Input: part model. Units: mm. Frame: model coordinates. A direction names the side the tool comes from. Coordinates: 2 decimals unless noted, no trailing zeros. Write each loop counter-clockwise with the first axis right and the second up, starting at its lowest first coordinate (ties: lowest second). Pieces come first, ordered by that corner, then holes. Notation, with made-up numbers: M -10.75,23.5 L 2.25,23.5 A16 cw 2.25,52.5 Z; hole C -26.5,-38 d6. An arc over 180 degrees is marked long. Write each question's results on one line, items separated by ' | '. Start each with the question number.
1. Section query B-B, the plane x = -105. Output: boundary loops of the cut face in (y, z), and give its area (3 significant figures).
2. Section query C-C, the plane y = 85. Output: boundary loops of the cut face in (x, z).
3. First-contact query: pin 1 (4 mm diameter, centred on x = 100.5, y = 92, fed in from +Z). Flat tip, straight axial feed; report the tip coordinate or a pass-through.
4. Section query A-A, the plane z = 89.5. Output: boundary loops of the cut face in (x, y).
5. Pull-direction query (X, two-part tool) for faces 3 (the flat face through (-96, -584, 127)), 4 (the flat face through (1219.2, -9, 63)), 5 (the flat face through (-16, 8, 25.4)), 6 (the flat face through (-1219.2, -9, 63)); classes: +X half, -X half, draft (parallel to the pull), parting line (faces both ways), or undercut.
6. Ray query, probe 1 along X at (y, z) = (248, 63); probe 2 along Y at (x, z) = (-781.5, 90.5); probe 3 along Z at (x, y) = (-842, 26). Return the intervals inside material, ascending.
7. Set-up query: faces 1 (the flat face through (-17, -660.4, 63)), 2 (the flat face through (-16, -558.8, 75)). Return all of +Z, -Z, +X, -X, +Y, -Y with unobstructed straight access to the full face (end or side cutting, diameter ignored); none if empty.
```python
from build123d import *

# Parameters (mm, degrees)
F0_W     = 2438.4
F0_H     = 1320.8
F0_W_2   = 2235.2
F0_H_2   = 1117.6
F1_DEPTH = 25.4
F2_W     = 2438.4
F2_H     = 1320.8
F2_W_2   = 2235.2
F2_H_2   = 1117.6
F3_DEPTH = 101.6


with BuildPart() as f1:
    # F0 (on Top) → F1 (new body)
    with BuildSketch(Plane.XY):
        Rectangle(F0_W, F0_H)
        Rectangle(F0_W_2, F0_H_2, mode=Mode.SUBTRACT)
        Rectangle(F0_W_2, F0_H_2)
    extrude(amount=F1_DEPTH)

    # F2 (on face) → F3 (join)
    with BuildSketch(Plane.XY.offset(25.4)):
        Rectangle(F2_W, F2_H)
        Rectangle(F2_W_2, F2_H_2, mode=Mode.SUBTRACT)
    extrude(amount=F3_DEPTH)


solid = f1.part
```
Answer:
1) outline: M -660.4,0 L 660.4,0 L 660.4,127 L 558.8,127 L 558.8,25.4 L -558.8,25.4 L -558.8,127 L -660.4,127 Z | area: 54,200 mm^2
2) outline: M -1219.2,0 L 1219.2,0 L 1219.2,127 L 1117.6,127 L 1117.6,25.4 L -1117.6,25.4 L -1117.6,127 L -1219.2,127 Z
3) pin 1: z = 25.4
4) outline: M -1219.2,-660.4 L 1219.2,-660.4 L 1219.2,660.4 L -1219.2,660.4 Z; hole M -1117.6,-558.8 L 1117.6,-558.8 L 1117.6,558.8 L -1117.6,558.8 Z
5) face 3: draft | face 4: +X half | face 5: undercut | face 6: -X half
6) probe 1: -1219.2 to -1117.6, 1117.6 to 1219.2 | probe 2: -660.4 to -558.8, 558.8 to 660.4 | probe 3: 0 to 25.4
7) face 1: +Z, -Z, +X, -X, -Y | face 2: +Z
